Can you work these out from the model? Positions are in its coordinate system, mm. Coordinates: 2 decimals unless noted, no trailing zeros. Order: outer loops, then holes, each group sorted by start corner. A loop starts at its lowest first (then second) coordinate and runs counter-clockwise, first axis right, second up. Notation, with made-up numbers: (-0.75, -30.75) -> (45.25, -30.75) arc R12 cw to (45.25, -9.75) -> close; hole circle Ø6 at (-2.5, -27.5). An arc over 180 degrees is marked (long way). Answer as a JSON object with one key per item and string values. Group by question number.
(1) I want a section at A-A, the plane x = 0. List the corners of the cut face in (y, z) for me (1 decimal).
(2) For pin 1 (1 mm diameter, centred on y = 42, z = 1, fed in from -X); pin 2 (11 mm diameter, centred on x = 40.46, y = 60.91, fed in from +Z) (3 decimals), each with a flat end and sliding along its axis, tell me the tip position at first contact or that it passes through.
(3) I need wall thicknesses on line 1 (Y direction, x = 0, z = 0.6); line 2 (X direction, y = 141, z = 1.9); line 3 (X direction, y = 2, z = 0.2). Which ranges of each line are inside material? Lowest first, please.
(4) I want a section at C-C, the plane y = 0. List the corners of the cut face in (x, z) for me (1 decimal).
(5) I want a section at D-D, the plane y = 82.5. List the corners of the cut face in (x, z) for me (3 decimals), plus the area to 3 significant figures.
(6) If we mould it in two halves opening along X, with no side actions, what happens to faces 1 (the cylindrical face through (-1.017, 7.744, 1.565)), 2 (the cylindrical face through (-50.623, 60.975, 1.565)), 3 (the cylindrical face through (50.623, 60.837, 1.565)), 4 (the cylindrical face through (42.272, 63.744, 1.565))? For each: pulls with the +X half, pulls with the -X half, needs draft (parallel to the pull), parting line crosses it, or undercut.
(7) I want a section at B-B, the plane z = 2.65. List the corners of the cut face in (x, y) for me, plus the area to 3 significant figures.
from build123d import *

# Parameters (mm, degrees)
SKETCH4_R           = 3.3655
SKETCH4_R_2         = 7.8105
SKETCH4_R_3         = 4.191
BOSS_EXTRUDE4_DEPTH = 3.175


with BuildPart() as part:
    # Sketch4 → Boss-Extrude4 (new body)
    # profile 1 of 3: a face of its own
    with BuildSketch(Plane.XY):
        with BuildLine():
            ThreePointArc((-10.16, 137.77468), (-9.863294022, 140.212103033), (-8.990505701, 142.507164257))
            Line((-8.990505701, 142.507164257), (-49.453246099, 65.638340515))
            ThreePointArc((-49.453246099, 65.638340515), (-50.622740399, 60.905856258), (-49.453246099, 56.173372001))
            Line((-49.453246099, 56.173372001), (-13.808489628, -2.118139324))
            ThreePointArc((-13.808489628, -2.118139324), (-13.929563886, -1.062144034), (-13.97, 0))
            Line((-13.97, 0), (-10.16, 137.77468))
        make_face()
        with Locations((-40.462740399, 60.905856258)):
            Circle(SKETCH4_R, mode=Mode.SUBTRACT)
    # profile 2 of 3: a face of its own
    with BuildSketch(Plane.XY):
        with BuildLine():
            ThreePointArc((49.453246099, 56.173372001), (50.622740399, 60.905856258), (49.453246099, 65.638340515))
            Line((49.453246099, 65.638340515), (8.990505701, 142.507164257))
            ThreePointArc((8.990505701, 142.507164257), (9.863294022, 140.212103033), (10.16, 137.77468))
            Line((10.16, 137.77468), (13.97, 0))
            ThreePointArc((13.97, 0), (13.929563886, -1.062144034), (13.808489628, -2.118139324))
            Line((13.808489628, -2.118139324), (49.453246099, 56.173372001))
        make_face()
        with Locations((40.462740399, 60.905856258)):
            Circle(SKETCH4_R, mode=Mode.SUBTRACT)
    # profile 3 of 3: a face of its own
    with BuildSketch(Plane.XY):
        with BuildLine():
            ThreePointArc((10.16, 137.77468), (9.863294022, 140.212103033), (8.990505701, 142.507164257))
            ThreePointArc((8.990505701, 142.507164257), (0, 147.93468), (-8.990505701, 142.507164257))
            ThreePointArc((-8.990505701, 142.507164257), (-9.863294022, 140.212103033), (-10.16, 137.77468))
            Line((-10.16, 137.77468), (-13.97, 0))
            ThreePointArc((-13.97, 0), (-13.929563886, -1.062144034), (-13.808489628, -2.118139324))
            Line((-13.808489628, -2.118139324), (-8.177790267, -11.326281223))
            ThreePointArc((-8.177790267, -11.326281223), (0, -13.97), (8.177790267, -11.326281223))
            Line((8.177790267, -11.326281223), (13.808489628, -2.118139324))
            ThreePointArc((13.808489628, -2.118139324), (13.929563886, -1.062144034), (13.97, 0))
            Line((13.97, 0), (10.16, 137.77468))
        make_face()
        Circle(SKETCH4_R_2, mode=Mode.SUBTRACT)
        with Locations((0, 137.77468)):
            Circle(SKETCH4_R_3, mode=Mode.SUBTRACT)
    extrude(amount=BOSS_EXTRUDE4_DEPTH)


solid = part.part
Computed values:
{
 "1": {"outline": "(-14, 0) -> (-7.8, 0) -> (-7.8, 3.2) -> (-14, 3.2) -> close; (7.8, 0) -> (133.6, 0) -> (133.6, 3.2) -> (7.8, 3.2) -> close; (142, 0) -> (147.9, 0) -> (147.9, 3.2) -> (142, 3.2) -> close"},
 "2": {"pin 1": "stops at x = -41.09", "pin 2": "stops at z = 3.175"},
 "3": {"line 1": "y = -13.97 to -7.81, 7.81 to 133.58, 141.97 to 147.93", "line 2": "x = -9.78 to -2.68, 2.68 to 9.78", "line 3": "x = -16.33 to -7.55, 7.55 to 16.33"},
 "4": {"outline": "(-15.1, 0) -> (-7.8, 0) -> (-7.8, 3.2) -> (-15.1, 3.2) -> close; (7.8, 0) -> (15.1, 0) -> (15.1, 3.2) -> (7.8, 3.2) -> close"},
 "5": {"outline": "(-40.577, 0) -> (40.577, 0) -> (40.577, 3.175) -> (-40.577, 3.175) -> close", "area": "258 mm2"},
 "6": {"face 1": "undercut", "face 2": "pulls with the -X half", "face 3": "pulls with the +X half", "face 4": "undercut"},
 "7": {"outline": "(-49.45, 56.17) -> (-8.18, -11.33) arc R13.97 ccw to (8.18, -11.33) -> (49.45, 56.17) arc R10.16 ccw to (49.45, 65.64) -> (8.99, 142.51) arc R10.16 ccw to (-8.99, 142.51) -> (-49.45, 65.64) arc R10.16 ccw to start; hole circle Ø6.73 at (-40.46, 60.91); hole circle Ø15.62 at (0, 0); hole circle Ø8.38 at (0, 137.77); hole circle Ø6.73 at (40.46, 60.91)", "area": "9,110 mm2"}
}
